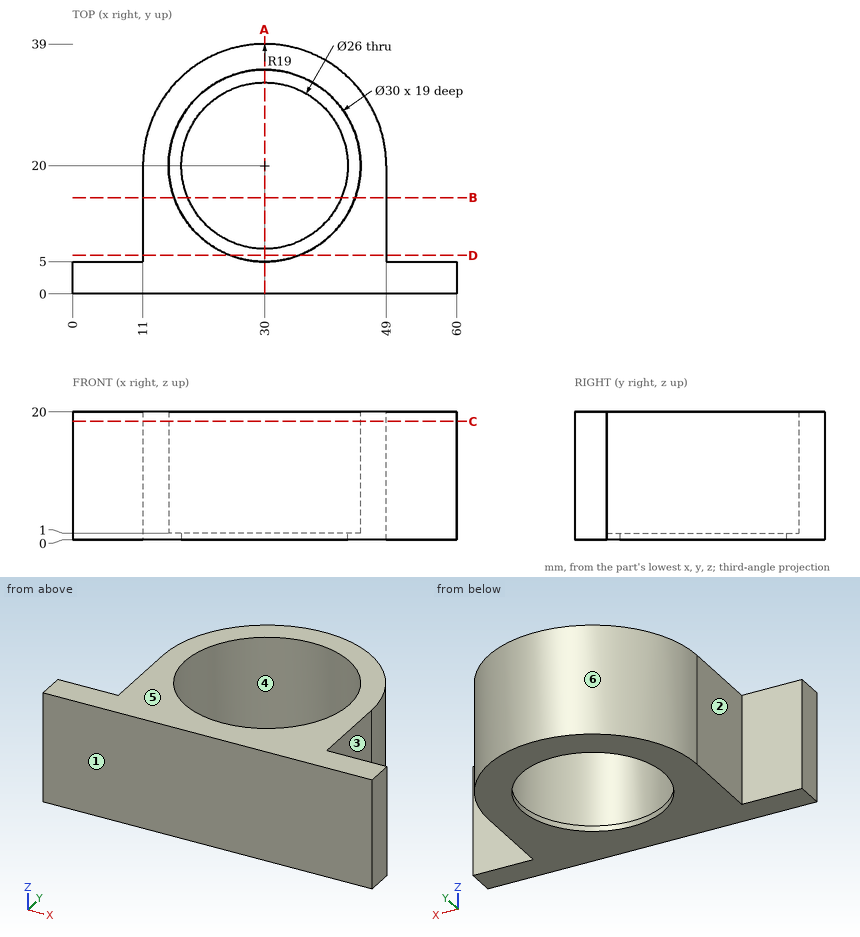
Answer from the drawing. Dimensions are ordinates in mm from the lowest x, y and z of the part. A direction names the side the tool comes from. Give positions to 0.01 mm unless a question says otherwise; leave off trailing zeros. Order: outer loops, then holes, each group sorted by start corner. A loop starts at its lowest first (then second) coordinate and runs counter-clockwise, first axis right, second up. Notation, with made-up numbers: (-28.5, 61.25) -> (1.5, 61.25) arc R25 cw to (1.5, 81.25) -> close; hole circle Ø6 at (-4.5, 13). An arc over 180 degrees is marked (long way). One line per item, written item: value. Start each with the question number.
(1) Straight lines are drawn through the part: L1, parallel to Y at x = 30, z = 15.75; L2, parallel to X at y = 20, z = 13.25; L3, parallel to Y at x = 30, z = 0.4. For each, find the intervals that lie inside material, in ascending order.
(2) A tool of negligible diameter and unlimited length cuts with its end or side. For the marked faces 1, 2 and 3, from which of +Z, -Z, +X, -X, +Y, -Y can it reach the whole face along a straight path? Write none if from no direction.
(3) The part is cut by section B-B (y = 15). Determine the outline of the cut face in (x, z).
(4) For a pull along Y with two mould halves and no side action, classify the marked faces 4, 5 and 6 as released by +Y, released by -Y, zero draft, split by the parting line, or undercut.
(5) The part is cut by section C-C (z = 18.5). Determine the outline of the cut face in (x, y), and give its area (3 significant figures).
(6) The part is cut by section D-D (y = 6). Determine the outline of the cut face in (x, z), and give its area (3 significant figures).
(7) The part is cut by section A-A (x = 30). Determine the outline of the cut face in (y, z).
(8) Flat-ended cylindrical pins translate along their axes: P1, Ø12, axis at x = 14.5, z = 4, coming from the +Y side; P2, Ø6, axis at x = 27.5, y = 31.5, coming from the -Z side; P3, Ø9, axis at x = 52, z = 8, coming from the +Y side; P4, Ø2, axis at x = 34, z = 8, coming from the +Y side. Find the tip coordinate at first contact, or state that the pin passes through.
Taken from the geometry:
1. L1: 0 to 5, 35 to 39
1. L2: 11 to 15, 45 to 49
1. L3: 0 to 7, 33 to 39
2. face 1: +Z, -Z, +X, -X, -Y
2. face 2: +Z, -Z, -X, +Y
2. face 3: +Z, -Z, +X, +Y
3. outline: (11, 0) -> (18, 0) -> (18, 1) -> (15.86, 1) -> (15.86, 20) -> (11, 20) -> close; (42, 0) -> (49, 0) -> (49, 20) -> (44.14, 20) -> (44.14, 1) -> (42, 1) -> close
4. face 4: undercut
4. face 5: zero draft
4. face 6: released by +Y
5. outline: (0, 0) -> (60, 0) -> (60, 5) -> (49, 5) -> (49, 20) arc R19 ccw to (11, 20) -> (11, 5) -> (0, 5) -> close; hole circle Ø30 at (30, 20)
5. area: 730 mm^2
6. outline: (11, 0) -> (49, 0) -> (49, 20) -> (35.39, 20) -> (35.39, 1) -> (24.61, 1) -> (24.61, 20) -> (11, 20) -> close
6. area: 555 mm^2
7. outline: (0, 0) -> (7, 0) -> (7, 1) -> (5, 1) -> (5, 20) -> (0, 20) -> close; (33, 0) -> (39, 0) -> (39, 20) -> (35, 20) -> (35, 1) -> (33, 1) -> close
8. P1: y = 36.45
8. P2: z = 0
8. P3: y = 27.4
8. P4: y = 38.76
